```python
from build123d import *
from build123d.topology import SkipClean

# Parameters (mm, degrees)
SKETCH1_W               = 200
SKETCH1_H               = 150
BOSS_EXTRUDE1_DEPTH     = 15
CUT_EXTRUDE2_DEPTH      = 30
SHELL2_T                = -3
SKETCH6_R               = 2.5
CUT_EXTRUDE3_DEPTH      = 30
CUT_EXTRUDE4_DEPTH      = 30
CUT_EXTRUDE4_DEPTH_BACK = 30
SKETCH7_R               = 5
CHAMFER1_SIZE           = 5
SKETCH8_R               = 2.5
CUT_EXTRUDE5_DEPTH      = 10
SKETCH9_W               = 105
SKETCH9_H               = 150
CUT_EXTRUDE8_DEPTH      = 50
SKETCH10_R              = 2.5
CUT_EXTRUDE9_DEPTH      = 50
SKETCH11_W              = 10
SKETCH11_H              = 2.828590786
CUT_EXTRUDE10_DEPTH     = 28
SKETCH12_W              = 10
SKETCH12_H              = 3.286754743
SKETCH12_H_2            = 3.432076944
CUT_EXTRUDE11_DEPTH     = 28


with BuildPart() as part:
    # Sketch1 → Boss-Extrude1 (new body)
    with BuildSketch(Plane.XY):
        Rectangle(SKETCH1_W, SKETCH1_H)
    extrude(amount=BOSS_EXTRUDE1_DEPTH)

    # Sketch5 → Cut-Extrude2 (cut)
    with BuildSketch(Plane(origin=(0, 0, 0), x_dir=(-1, 0, 0), z_dir=(0, 0, -1))):
        with BuildLine():
            Line((100, 75), (5, 75))
            ThreePointArc((5, 75), (24.038059223, 29.038059223), (70, 10))
            Line((70, 10), (100, 10))
            Line((100, 10), (100, 75))
        make_face()
        with BuildLine():
            ThreePointArc((70, -10), (24.038059223, -29.038059223), (5, -75))
            Line((5, -75), (100, -75))
            Line((100, -75), (100, -10))
            Line((100, -10), (70, -10))
        make_face()
        with BuildLine():
            Line((-80, -10), (-100, -10))
            Line((-100, -10), (-100, -75))
            Line((-100, -75), (-15, -75))
            ThreePointArc((-15, -75), (-34.038059223, -29.038059223), (-80, -10))
        make_face()
        with BuildLine():
            Line((-100, 75), (-100, 10))
            Line((-100, 10), (-80, 10))
            ThreePointArc((-80, 10), (-34.038059223, 29.038059223), (-15, 75))
            Line((-15, 75), (-100, 75))
        make_face()
    extrude(amount=-CUT_EXTRUDE2_DEPTH, mode=Mode.SUBTRACT)

    # Shell2
    shell2_openings = [part.faces().sort_by_distance(p)[0] for p in [
        (3.044348512, 0, 15),
    ]]
    offset(amount=SHELL2_T, openings=shell2_openings, kind=Kind.INTERSECTION)

    # Sketch6 → Cut-Extrude3 (cut)
    with BuildSketch(Plane(origin=(0, 0, 0), x_dir=(-1, 0, 0), z_dir=(0, 0, -1))):
        with Locations((-5, 65)):
            Circle(SKETCH6_R)
        with Locations((-5, -65)):
            Circle(SKETCH6_R)
    extrude(amount=-CUT_EXTRUDE3_DEPTH, mode=Mode.SUBTRACT)

    # Sketch7 → Cut-Extrude4 (cut, two sides: drawn at the far end of the back side and taken through both)
    with BuildSketch(Plane(origin=(0, 0, 0), x_dir=(1, 0, 0), z_dir=(0, 1, 0)).offset(-CUT_EXTRUDE4_DEPTH_BACK)):
        with Locations((-80, -15)):
            Circle(SKETCH7_R)
        with Locations((80, -15)):
            Circle(SKETCH7_R)
    extrude(amount=CUT_EXTRUDE4_DEPTH + CUT_EXTRUDE4_DEPTH_BACK, mode=Mode.SUBTRACT)

    # Chamfer1
    chamfer1_edges = [part.edges().sort_by_distance(p)[0] for p in [
        (-100, 0, 0),
        (5, 75, 0),
        (100, 0, 0),
        (5, -75, 0),
        (90, 10, 0),
        (34.038059223, 29.038059223, 0),
        (34.038059223, -29.038059223, 0),
        (90, -10, 0),
        (-24.038059223, -29.038059223, 0),
        (-85, -10, 0),
        (-24.038059223, 29.038059223, 0),
        (-85, 10, 0),
    ]]
    chamfer(chamfer1_edges, length=CHAMFER1_SIZE)

    # Sketch8 → Cut-Extrude5 (cut)
    with BuildSketch(Plane.XY.offset(3)):
        with Locations((-22, 15)):
            Circle(SKETCH8_R)
        with Locations((-22, -15)):
            Circle(SKETCH8_R)
    extrude(amount=-CUT_EXTRUDE5_DEPTH, mode=Mode.SUBTRACT)

    # Sketch9 → Cut-Extrude8 (cut)
    with BuildSketch(Plane.XY):
        with Locations((-47.5, 0)):
            Rectangle(SKETCH9_W, SKETCH9_H)
    extrude(amount=CUT_EXTRUDE8_DEPTH, mode=Mode.SUBTRACT)

    # Mirror4: part across plane


with BuildPart() as part_1:
    with SkipClean():  # the faces are left unmerged after this step: merging them gives an invalid solid
        add(part.part)
        add(part.part.mirror(Plane(origin=(5, 75, 50), x_dir=(0, 0, 1), z_dir=(-1, 0, 0))))

    # Sketch10 → Cut-Extrude9 (cut)
    with SkipClean():  # the faces are left unmerged after this step: merging them gives an invalid solid
        with BuildSketch(Plane.XY):
            with Locations((-14.2, 15)):
                Circle(SKETCH10_R)
            with Locations((-14.2, -15)):
                Circle(SKETCH10_R)
        extrude(amount=CUT_EXTRUDE9_DEPTH, mode=Mode.SUBTRACT)

    # Sketch11 → Cut-Extrude10 (cut)
    with SkipClean():  # the faces are left unmerged after this step: merging them gives an invalid solid
        with BuildSketch(Plane.ZY.offset(90)):
            with Locations((10, 11.414295393)):
                Rectangle(SKETCH11_W, SKETCH11_H)
            with Locations((10, -11.414295393)):
                Rectangle(SKETCH11_W, SKETCH11_H)
        extrude(amount=-CUT_EXTRUDE10_DEPTH, mode=Mode.SUBTRACT)

    # Sketch12 → Cut-Extrude11 (cut)
    with SkipClean():  # the faces are left unmerged after this step: merging them gives an invalid solid
        with BuildSketch(Plane(origin=(100, 0, 0), x_dir=(0, 0, -1), z_dir=(1, 0, 0))):
            with Locations((-10, -11.643377372)):
                Rectangle(SKETCH12_W, SKETCH12_H)
            with Locations((-10, 11.716038472)):
                Rectangle(SKETCH12_W, SKETCH12_H_2)
        extrude(amount=-CUT_EXTRUDE11_DEPTH, mode=Mode.SUBTRACT)


solid = part_1.part
```
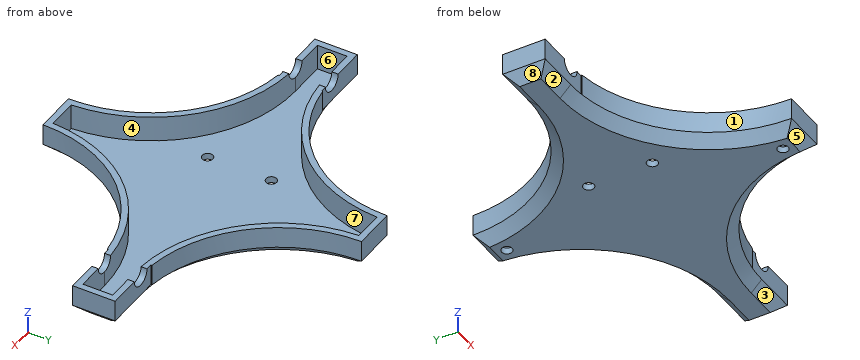
Geometry check sheet. Reference: the model listing, model coordinates, mm. Face numbers are marked on the shaded views. A direction names the side the tool comes from. Coordinates: 2 decimals unless noted, no trailing zeros. Order: outer loops, then holes, each group sorted by start corner. A loop starts at its lowest first (then second) coordinate and runs counter-clockwise, first axis right, second up.
Q1. Thickness scan on probe 1 along Y at (x, z) = (85.5, 11.5); probe 2 along Y at (x, z) = (-14.2, 2.45); probe 3 along Y at (x, z) = (-14.2, 1.3). Record the ranges inside material, lowest first.
Reply:
probe 1: y = -10 to -7, 7 to 10
probe 2: y = -36.93 to -17.5, -12.5 to 12.5, 17.5 to 36.93
probe 3: y = -34.92 to -17.5, -12.5 to 12.5, 17.5 to 34.92
Q2. Sectioned sample at A-A on z = 7.5. Record the cut outline in (x, y), and give its area (3 significant figures).
Reply:
outline: (-90, -10) - (-62, -10) - (-62, -10.49) arc R65 cw to (-5, -75) - (15, -75) arc R65 cw to (72, -10.49) - (72, -10) - (100, -10) - (100, 10) - (72, 10) - (72, 10.49) arc R65 cw to (15, 75) - (-5, 75) arc R65 cw to (-62, 10.49) - (-62, 10) - (-90, 10) - close; hole (-87, -7) - (-70, -7) arc R68 cw to (-2.07, -72) - (12.07, -72) arc R68 cw to (80, -7) - (97, -7) - (97, 7) - (80, 7) arc R68 cw to (12.07, 72) - (-2.07, 72) arc R68 cw to (-70, 7) - (-87, 7) - close
area: 1,660 mm2
Q3. Tool access check on the marked faces 1, 2, 3 and 4. Record the directions out of +Z, -Z, +X, -X, +Y, -Y that give a thin tool (end or side, any length) a straight path to the whole face; none if there is none.
Reply:
face 1: +Z, -Z, -X, -Y
face 2: -Z, -X, -Y
face 3: -Z, +X, -Y
face 4: +Z
Q4. Sectioned sample at C-C on x = -14.2. Give the number of separate pieces and of enclosed holes in the cut face, and give its area (3 significant figures).
Reply:
separate pieces: 3
enclosed holes: 0
area: 307 mm2
Q5. Depth check by flat-ended pin: pin 1 Ø1.5 at (x, z) = (52.5, 3.5) entering from +Y; pin 2 Ø6 at (x, z) = (-46, 7.5) entering from +Y; pin 3 Ø2 at (y, z) = (-25.5, 8) entering from +X; pin 4 Ø6 at (x, y) = (-12, 59) entering from -Z. Enter the tip coordinate at first touch or a pass-through.
Reply:
pin 1: stops at y = 15.35
pin 2: stops at y = 15.87
pin 3: stops at x = 39.08
pin 4: passes through
Q6. Draft check along X on the marked faces 5, 6, 7 and 8. Enter one of: released by +X, released by -X, zero draft, split by the parting line, or undercut.
Reply:
face 5: zero draft
face 6: undercut
face 7: undercut
face 8: released by -X
Q7. Sectioned sample at B-B on y = 1.5. Record the cut outline in (x, z), and give its area (3 significant figures).
Reply:
outline: (-90, 5) - (-85, 0) - (95, 0) - (100, 5) - (100, 15) - (97, 15) - (97, 3) - (-87, 3) - (-87, 15) - (-90, 15) - close
area: 617 mm2
